Design review of the part built by this model. Coordinates are the model's own, in mm. A direction names the side the tool comes from. Coordinates: 2 decimals unless noted, no trailing zeros. Loops run counter-clockwise (first coordinate to the right, second up) from the corner with the lowest first, then second, coordinate; pieces in that order, holes last.
Q1. Add section C-C on x = 3.25. Give the boundary of the cut face in (y, z).
Q2. Add section D-D on z = 1. Give the boundary of the cut face in (x, y).
Q3. Wall thickness on probe 1 along Z at (x, y) = (-3, 0.25); probe 2 along X at (y, z) = (-0.75, 2.5); probe 3 along X at (y, z) = (-1, -5): over which ranges is each line inside the solid? List them lowest first.
Q4. Draft analysis for pull direction Y (two halves, no side actions). For faces 1 (the face through (0, -2, -3)), 2 (the face through (2, -2, 0)), 3 (the face through (-1.498, -0.082, 3.014)), state which applies: released by +Y, released by -Y, zero draft, split by the parting line, or undercut.
Q5. Add section A-A on z = -3.5. Give the boundary of the cut face in (x, y).
Q6. For P1, Ø1.5, axis at x = -2.5, z = -2.5, coming from the +Y side; P2, Ø2, axis at x = 2, z = -4, coming from the +Y side; P3, Ø3, axis at y = -0.5, z = -4, coming from the -X side, all flat-tipped, find the tip position at first contact; note any pin that passes through.
Q7. Add section B-B on y = 0. Give the boundary of the cut face in (x, z), and give its area (3 significant figures).
Q8. Machinability: for faces 4 (the face through (0.82, -1.256, 3.014)), 5 (the face through (0, 0, -6)), which of the approach directions +Z, -Z, +X, -X, +Y, -Y give a long, thin tool a straight path to every point of the face, cutting with its end or side? Answer none if there is none.
```python
from build123d import *

# Parameters (mm, degrees)
SKETCH_1_R          = 3.5
EXTRUDE_1_DEPTH     = 4
CUT_EXTRUDE_1_DEPTH = 2
SKETCH_3_R          = 2
EXTRUDE_2_DEPTH     = 6


with BuildPart() as part:
    # 草图1 → 凸台-拉伸1 (new body)
    with BuildSketch(Plane.XY):
        Circle(SKETCH_1_R)
    extrude(amount=EXTRUDE_1_DEPTH)

    # 草图2 → 切除-拉伸1 (cut)
    with BuildSketch(Plane.XY.offset(4)):
        Polygon((1.551335969, -0.77029651), (1.44276433, 0.958348104), (-0.108571638, 1.728644613), (-1.551335969, 0.77029651), (-1.44276433, -0.958348104), (0.108571638, -1.728644613), align=None)
    extrude(amount=-CUT_EXTRUDE_1_DEPTH, mode=Mode.SUBTRACT)

    # 草图3 → 凸台-拉伸2 (add)
    with BuildSketch(Plane(origin=(0, 0, 0), x_dir=(-1, 0, 0), z_dir=(0, 0, -1))):
        Circle(SKETCH_3_R)
    extrude(amount=EXTRUDE_2_DEPTH)


solid = part.part
```
Entries:
1. outline: (-1.3, 0) - (1.3, 0) - (1.3, 4) - (-1.3, 4) - close
2. outline: circle Ø7 at (0, 0)
3. probe 1: z = 0 to 4
3. probe 2: x = -3.42 to -1.46, 1.55 to 3.42
3. probe 3: x = -1.73 to 1.73
4. face 1: split by the parting line
4. face 2: zero draft
4. face 3: undercut
5. outline: circle Ø4 at (0, 0)
6. P1: stops at y = 0.97
6. P2: stops at y = 1.73
6. P3: stops at x = -2
7. outline: (-3.5, 0) - (-2, 0) - (-2, -6) - (2, -6) - (2, 0) - (3.5, 0) - (3.5, 4) - (1.5, 4) - (1.5, 2) - (-1.5, 2) - (-1.5, 4) - (-3.5, 4) - close
7. area: 46.0 mm2
8. face 4: +Z
8. face 5: -Z, +X, -X, +Y, -Y
